Here's how the part is built. I have some questions about the finished solid (model axes, mm). Face numbers are marked on the shaded views. Round coordinates to 2 decimals unless told otherwise and drop trailing zeros. Loops run counter-clockwise (first coordinate to the right, second up) from the corner with the lowest first, then second, coordinate; pieces in that order, holes last. Notation, with made-up numbers: M -28,89.5 L -22,89.5 A11 cw -22,104.5 Z; hole C -31,-28 d3. An arc over 180 degrees is marked long. Answer as a JSON object with one key per item and string values.
from build123d import *

# Parameters (mm, degrees)
F0_R     = 10.5
F1_DEPTH = 6.35
F2_R     = 0.0508


with BuildPart() as f1:
    # F0 (on Top) → F1 (new body)
    with BuildSketch(Plane.XY):
        with BuildLine():
            ThreePointArc((-35.850693, 5.992529), (-15.4911, 0), (-35.850693, -5.992529))
            ThreePointArc((-35.850693, -5.992529), (-25.708936, -25.695003), (-6.011962, -35.847439))
            ThreePointArc((-6.011962, -35.847439), (0, -15.50641), (6.011962, -35.847439))
            ThreePointArc((6.011962, -35.847439), (25.708936, -25.695003), (35.850693, -5.992529))
            ThreePointArc((35.850693, -5.992529), (15.4911, 0), (35.850693, 5.992529))
            ThreePointArc((35.850693, 5.992529), (25.708936, 25.695003), (6.011962, 35.847439))
            ThreePointArc((6.011962, 35.847439), (0, 15.50641), (-6.011962, 35.847439))
            ThreePointArc((-6.011962, 35.847439), (-25.708936, 25.695003), (-35.850693, 5.992529))
        make_face()
        Circle(F0_R, mode=Mode.SUBTRACT)
    extrude(amount=F1_DEPTH)

    # F2
    f2_edges = [f1.edges().sort_by_distance(p)[0] for p in [
        (-25.708936, 25.695003, 0),
        (25.708936, 25.695003, 0),
        (25.708936, -25.695003, 0),
        (0, -15.50641, 0),
        (15.4911, 0, 0),
        (0, 15.50641, 0),
        (-15.4911, 0, 0),
        (-25.708936, -25.695003, 0),
        (-25.708936, -25.695003, 6.35),
        (-25.708936, 25.695003, 6.35),
        (25.708936, 25.695003, 6.35),
        (15.4911, 0, 6.35),
        (0, 15.50641, 6.35),
        (-15.4911, 0, 6.35),
        (0, -15.50641, 6.35),
        (25.708936, -25.695003, 6.35),
    ]]
    fillet(f2_edges, radius=F2_R)


solid = f1.part
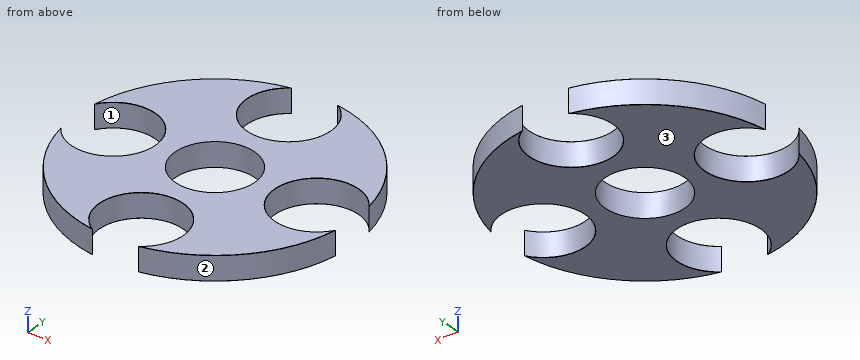
Item 1: I want a section at B-B on y = 0. List the corners of the cut face in (x, z) for me, plus the area to 3 significant figures.
Solution:
{"outline": "M -15.49,0.05 A0.05 ccw -15.44,0 L -10.5,0 L -10.5,6.35 L -15.44,6.35 A0.05 ccw -15.49,6.3 Z; M 10.5,0 L 15.44,0 A0.05 ccw 15.49,0.05 L 15.49,6.3 A0.05 ccw 15.44,6.35 L 10.5,6.35 Z", "area": "63.4 mm2"}
Item 2: I want a section at C-C on z = 3.25. List the corners of the cut face in (x, y) for me.
Solution:
{"outline": "M -35.85,-5.99 A36.35 ccw -6.01,-35.85 A11.06 cw long 6.01,-35.85 A36.35 ccw 35.85,-5.99 A11.06 cw long 35.85,5.99 A36.35 ccw 6.01,35.85 A11.06 cw long -6.01,35.85 A36.35 ccw -35.85,5.99 A11.06 cw long Z; hole C 0,0 d21"}
Item 3: I want a section at A-A on x = 0. List the corners of the cut face in (y, z) for me, plus the area to 3 significant figures.
Solution:
{"outline": "M -15.51,0.05 A0.05 ccw -15.46,0 L -10.5,0 L -10.5,6.35 L -15.46,6.35 A0.05 ccw -15.51,6.3 Z; M 10.5,0 L 15.46,0 A0.05 ccw 15.51,0.05 L 15.51,6.3 A0.05 ccw 15.46,6.35 L 10.5,6.35 Z", "area": "63.6 mm2"}
Item 4: If I drill on L1, parallel to Y at x = -9.5, z = 5; L2, parallel to X at y = -9, z = 6.25; L3, parallel to X at y = -0.5, z = 5, over which ranges is the centre line in solid material (lowest first)? Write a range as from..to.
Solution:
{"L1": "y = -35.08..-32.23, -20.9..-4.47, 4.47..20.9, 32.23..35.08", "L2": "x = -35.22..-32.98, -20.12..-5.41, 5.41..20.12, 32.98..35.22", "L3": "x = -15.5..-10.49, 10.49..15.5"}
Item 5: We'd pull the mould along X, two halves only. Please class the marked faces 1, 2 and 3: +X half, -X half, draft (parallel to the pull), parting line (faces both ways), or undercut.
Solution:
{"face 1": "undercut", "face 2": "+X half", "face 3": "draft"}
Item 6: For P1, Ø5, axis at x = 6, y = -1.5, coming from the -Z side; P2, Ø2, axis at y = 2, z = 1, coming from the +X side; P3, Ø3, axis at y = -9.5, z = 2, coming from the -X side, each with a flat end and sliding along its axis, tell me the tip position at first contact or that it passes through.
Solution:
{"P1": "passes through", "P2": "stops at x = 15.91", "P3": "stops at x = -35.46"}
